```python
from build123d import *

# Parameters (mm, degrees)
SKETCH1_W           = 50
SKETCH1_H           = 70
BOSS_EXTRUDE1_DEPTH = 1.5
FILLET1_R           = 10


with BuildPart() as part:
    # Sketch1 → Boss-Extrude1 (new body)
    with BuildSketch(Plane.XY):
        Rectangle(SKETCH1_W, SKETCH1_H)
        with BuildLine():
            Line((-3, -29.653280585), (-3, 29.653280585))
            ThreePointArc((-3, 29.653280585), (0, 32.653280585), (3, 29.653280585))
            Line((3, 29.653280585), (3, -29.653280585))
            ThreePointArc((3, -29.653280585), (0, -32.653280585), (-3, -29.653280585))
        make_face(mode=Mode.SUBTRACT)
    extrude(amount=BOSS_EXTRUDE1_DEPTH)

    # Fillet1
    fillet1_edges = [part.edges().sort_by_distance(p)[0] for p in [
        (-25, 35, 0.75),
        (25, 35, 0.75),
    ]]
    fillet(fillet1_edges, radius=FILLET1_R)


solid = part.part
```
CAD build for the part. Positions are in the model's coordinates, mm. A direction names the side the tool comes from. Coordinates: 2 decimals unless noted, no trailing zeros. Order: outer loops, then holes, each group sorted by start corner. A loop starts at its lowest first (then second) coordinate and runs counter-clockwise, first axis right, second up. Notation, with made-up numbers: (51, 74.5) - (81, 74.5) arc R14 cw to (81, 90.5) - close; hole circle Ø7 at (-5.5, 24). An arc over 180 degrees is marked (long way). Use a Markdown table: item, result. Add a question column.
(1) Saw through at C-C (y = 8). Give the cut face in (x, z), then the cut area to 3 significant figures.
(2) Pull direction X, two halves, no side cores. Call faces 3 (the face through (-0.066, 32.653, 0.74)), 4 (the face through (-22.15, 31.99, 0.76)), 5 (the face through (21.99, 32.15, 0.76)): +X half, -X half, draft (parallel to the pull), parting line (faces both ways), or undercut.
(3) Which spindle directions (+Z, -Z, +X, -X, +Y, -Y) get a long thin tool onto all of the face, cutting with end or side? Do faces 1 (the face through (0.066, -32.653, 0.74)), 2 (the face through (5, 0, 1.5)). Say none if no direction does.
(4) Saw through at A-A (x = 0). Give the cut face in (y, z), then the cut area to 3 significant figures.
(5) Drill centre lines: line 1 along X through (y, z) = (-1.5, 0.95); line 2 along X through (y, z) = (31, 0.5); line 3 along Y through (x, z) = (-19.5, 1). Where is each one in solid material? Low to high. Write a range as [from, to].
(6) Saw through at B-B (z = 1.1). Give the cut face in (x, y), then the cut area to 3 significant figures.
Solved:
| question | item | result |
|---|---|---|
| 1 | outline | (-25, 0) - (-3, 0) - (-3, 1.5) - (-25, 1.5) - close; (3, 0) - (25, 0) - (25, 1.5) - (3, 1.5) - close |
| 1 | area | 66.0 mm² |
| 2 | face 3 | undercut |
| 2 | face 4 | -X half |
| 2 | face 5 | +X half |
| 3 | face 1 | +Z, -Z |
| 3 | face 2 | +Z, +X, -X, +Y, -Y |
| 4 | outline | (-35, 0) - (-32.65, 0) - (-32.65, 1.5) - (-35, 1.5) - close; (32.65, 0) - (35, 0) - (35, 1.5) - (32.65, 1.5) - close |
| 4 | area | 7.04 mm² |
| 5 | line 1 | x = [-25, -3], [3, 25] |
| 5 | line 2 | x = [-23, -2.68], [2.68, 23] |
| 5 | line 3 | y = [-35, 33.93] |
| 6 | outline | (-25, -35) - (25, -35) - (25, 25) arc R10 ccw to (15, 35) - (-15, 35) arc R10 ccw to (-25, 25) - close; hole (-3, -29.65) arc R3 ccw to (3, -29.65) - (3, 29.65) arc R3 ccw to (-3, 29.65) - close |
| 6 | area | 3,070 mm² |
